from build123d import *

# Parameters (mm, degrees)
SKETCH5_W           = 190
SKETCH5_H           = 36
BOSS_EXTRUDE1_DEPTH = 8
SKETCH6_R           = 13
SKETCH6_R_2         = 12.99768992
CUT_EXTRUDE1_DEPTH  = 6
BOSS_EXTRUDE2_DEPTH = 116
FILLET1_R           = 10


with BuildPart() as part:
    # Sketch5 → Boss-Extrude1 (new body)
    with BuildSketch(Plane(origin=(0, 0, 0), x_dir=(1, 0, 0), z_dir=(0, 1, 0))):
        with Locations((95, 18)):
            Rectangle(SKETCH5_W, SKETCH5_H)
    extrude(amount=BOSS_EXTRUDE1_DEPTH)

    # Sketch6 → Cut-Extrude1 (cut)
    with BuildSketch(Plane(origin=(0, 8, 0), x_dir=(1, 0, 0), z_dir=(0, 1, 0))):
        with Locations(Location((23, 18, 0), (0, 0, 270))):
            Circle(SKETCH6_R)
        with Locations(Location((59, 18, 0), (0, 0, 270))):
            Circle(SKETCH6_R)
        with Locations(Location((95.004620161, 18, 0), (0, 0, 270))):
            Circle(SKETCH6_R)
        with Locations(Location((131.004620161, 18, 0), (0, 0, 270))):
            Circle(SKETCH6_R)
        with Locations(Location((167.00231008, 18, 0), (0, 0, 270))):
            Circle(SKETCH6_R_2)
    extrude(amount=-CUT_EXTRUDE1_DEPTH, mode=Mode.SUBTRACT)

    # Sketch7 → Boss-Extrude2 (add)
    with BuildSketch(Plane(origin=(0, 8, 0), x_dir=(1, 0, 0), z_dir=(0, 1, 0))):
        with BuildLine():
            Line((0, 0), (10, 0))
            Line((10, 0), (10, 8))
            ThreePointArc((10, 8), (8.585786438, 8.585786438), (8, 10))
            Line((8, 10), (0, 10))
            Line((0, 10), (0, 0))
        make_face()
        with BuildLine():
            Line((0, 36), (10, 36))
            Line((10, 36), (10, 28))
            ThreePointArc((10, 28), (8.585786438, 27.414213562), (8, 26))
            Line((8, 26), (0, 26))
            Line((0, 26), (0, 36))
        make_face()
        with BuildLine():
            Line((190, 36), (180, 36))
            Line((180, 36), (180, 28))
            ThreePointArc((180, 28), (181.414213562, 27.414213562), (182, 26))
            Line((182, 26), (190, 26))
            Line((190, 26), (190, 36))
        make_face()
        with BuildLine():
            Line((190, 0), (180, 0))
            Line((180, 0), (180, 8))
            ThreePointArc((180, 8), (181.414213562, 8.585786438), (182, 10))
            Line((182, 10), (190, 10))
            Line((190, 10), (190, 0))
        make_face()
    extrude(amount=BOSS_EXTRUDE2_DEPTH)

    # Fillet1
    fillet1_edges = [part.edges().sort_by_distance(p)[0] for p in [
        (190, 62, 0),
        (190, 62, -36),
        (0, 62, -36),
        (0, 62, 0),
    ]]
    fillet(fillet1_edges, radius=FILLET1_R - 0.0001)  # a hair under: the kernel refuses the full size


solid = part.part
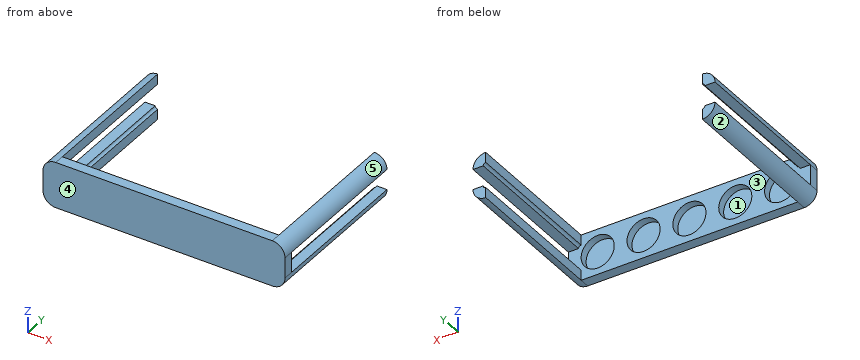
Could you check a few things on this model? Use its own coordinates, in mm. Face numbers are marked on the shaded views. A direction names the side the tool comes from. Coordinates: 2 decimals unless noted, no trailing zeros. Loops run counter-clockwise (first coordinate to the right, second up) from the corner with the lowest first, then second, coordinate; pieces in that order, holes last.
1. We'd pull the mould along X, two halves only. Please class the marked faces 3, 4 and 5: released by +X, released by -X, zero draft, split by the parting line, or undercut.
2. I need wall thicknesses on L1, parallel to X at y = 4, z = -18; L2, parallel to Y at x = 25, z = -12.5; L3, parallel to Y at x = 11.5, z = -8. Which ranges of each line are inside material? Lowest first, please.
3. Imagine slicing it at C-C (z = -16). Please give me the cut outline in (x, y).
4. Imagine slicing it at B-B (x = 59). Please give me the cut outline in (y, z).
5. Imagine slicing it at A-A (y = 19). Give the number of separate pieces and of enclosed holes in the cut face, and give its area (3 significant figures).
6. Imagine slicing it at D-D (x = 15). Please give me the cut outline in (y, z).
7. For P1, Ø9, axis at y = 73.5, z = -3, coming from the +X side; P2, Ø6.5, axis at x = 5.5, y = 74.5, coming from the +Z side; P3, Ø4, axis at x = 167.5, z = -19, coming from the +Y side; P4, Ø6, axis at x = 103.5, z = -6, coming from the -Y side, each with a flat end and sliding along its axis, tell me the tip position at first contact or that it passes through.
8. For the marked faces 1 and 2, which set-ups out of +Z, -Z, +X, -X, +Y, -Y let a thin tool reach every point of the face, with its end or its side?
Computed values:
1. face 3: undercut
1. face 4: zero draft
1. face 5: released by +X
2. L1: x = 0 to 10, 36 to 46, 72 to 82, 108 to 118, 144 to 154, 180 to 190
2. L2: y = 0 to 2
2. L3: y = 0 to 8
3. outline: (0, 0) - (190, 0) - (190, 8) - (179.85, 8) - (179.85, 2) - (154.16, 2) - (154.16, 8) - (143.85, 8) - (143.85, 2) - (118.16, 2) - (118.16, 8) - (107.85, 8) - (107.85, 2) - (82.16, 2) - (82.16, 8) - (71.85, 8) - (71.85, 2) - (46.15, 2) - (46.15, 8) - (35.85, 8) - (35.85, 2) - (10.15, 2) - (10.15, 8) - (0, 8) - close
4. outline: (0, -36) - (8, -36) - (8, -31) - (2, -31) - (2, -5) - (8, -5) - (8, 0) - (0, 0) - close
5. separate pieces: 4
5. enclosed holes: 0
5. area: 302 mm2
6. outline: (0, -36) - (8, -36) - (8, -28.25) - (2, -28.25) - (2, -7.75) - (8, -7.75) - (8, 0) - (0, 0) - close
7. P1: stops at x = 189.68
7. P2: stops at z = -0.08
7. P3: stops at y = 2
7. P4: stops at y = 0
8. face 1: +Y
8. face 2: -Z, -X, +Y, -Y
